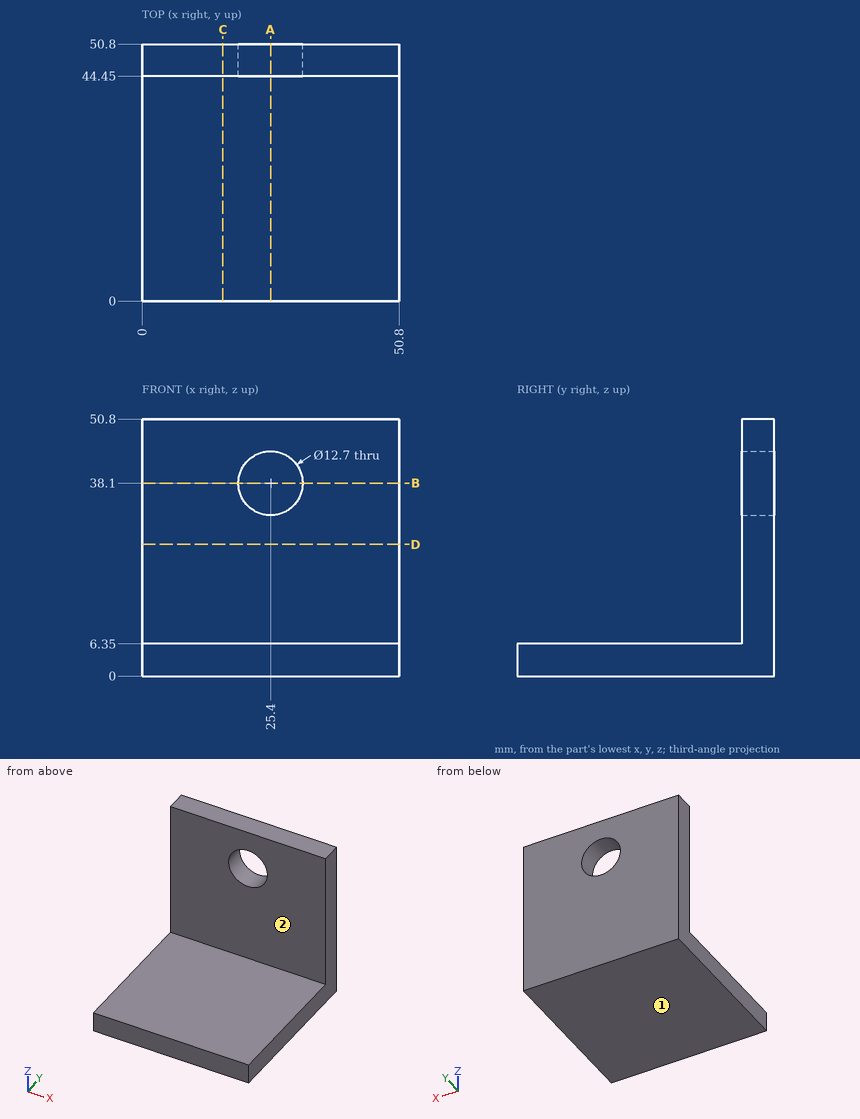
Geometry check sheet. Reference: drawing and pictorial views, mm from the part's lowest x, y, z. A direction names the side the tool comes from. Coordinates: 2 decimals unless noted, no trailing zeros. Order: outer loops, then holes, each group sorted by start corner. A loop starts at its lowest first (then second) coordinate and runs counter-clockwise, first axis right, second up.
1. Sectioned sample at A-A, the plane x = 25.4. Record the cut outline in (y, z), and give its area (3 significant figures).
Results found:
outline: (0, 0) - (50.8, 0) - (50.8, 31.75) - (44.45, 31.75) - (44.45, 6.35) - (0, 6.35) - close; (44.45, 44.45) - (50.8, 44.45) - (50.8, 50.8) - (44.45, 50.8) - close
area: 524 mm2
2. Sectioned sample at D-D, the plane z = 26. Record the cut outline in (x, y).
Results found:
outline: (0, 44.45) - (50.8, 44.45) - (50.8, 50.8) - (0, 50.8) - close
3. Scan lines: line 1 (Z direction, x = 25.4, y = 46.5); line 2 (Z direction, x = 21, y = 32); line 3 (Y direction, x = 14, z = 24.5). Record each from-to range of solid material in increasing order.
Results found:
line 1: z = 0 to 31.75, 44.45 to 50.8
line 2: z = 0 to 6.35
line 3: y = 44.45 to 50.8
4. Go/stop test with flat-tipped pins: pin 1 Ø14.5 at (x, z) = (25.4, 38.1) entering from +Y; pin 2 Ø2 at (x, y) = (9.5, 17.5) entering from +Z; pin 3 Ø13.5 at (x, z) = (19.5, 38.5) entering from -Y. Record where each tip stops, or that it passes through.
Results found:
pin 1: stops at y = 50.8
pin 2: stops at z = 6.35
pin 3: stops at y = 44.45
5. Sectioned sample at B-B, the plane z = 38.1. Record the cut outline in (x, y), and give its area (3 significant figures).
Results found:
outline: (0, 44.45) - (19.05, 44.45) - (19.05, 50.8) - (0, 50.8) - close; (31.75, 44.45) - (50.8, 44.45) - (50.8, 50.8) - (31.75, 50.8) - close
area: 242 mm2
6. Sectioned sample at C-C, the plane x = 16. Record the cut outline in (y, z), and give its area (3 significant figures).
Results found:
outline: (0, 0) - (50.8, 0) - (50.8, 50.8) - (44.45, 50.8) - (44.45, 6.35) - (0, 6.35) - close
area: 605 mm2
7. Set-up check for the marked faces 1 and 2: record each of +Z, -Z, +X, -X, +Y, -Y from which the full face is reachable in a straight line by a thin tool's end or side.
Results found:
face 1: -Z, +X, -X, +Y, -Y
face 2: +Z, +X, -X, -Y
